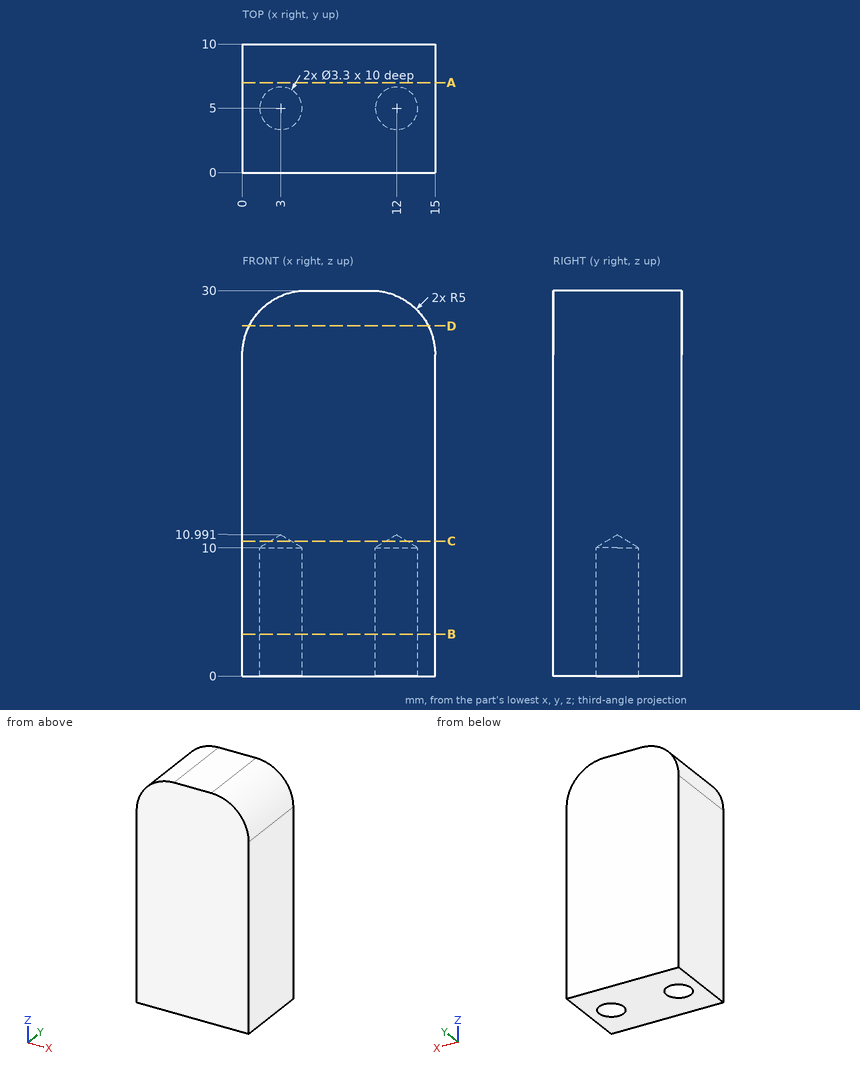
Source: three-view drawing plus pictorial views. Frame: mm from the lowest corner of the part. Coordinates: 2 decimals unless noted, no trailing zeros. Order: outer loops, then holes, each group sorted by start corner. A loop starts at its lowest first (then second) coordinate and runs counter-clockwise, first axis right, second up. Notation, with made-up numbers: (46.25, -27.75) -> (75.25, -27.75) arc R15 ccw to (75.25, -22.75) -> close; hole circle Ø11 at (0.5, 28.5). An arc over 180 degrees is marked (long way). Write item = value, one per line.
(1) Cut plane D-D on z = 27.25. Return loops of the section in (x, y) (1 decimal), plus the area to 3 significant figures.
Solved:
outline = (0.5, 0) -> (14.5, 0) -> (14.5, 10) -> (0.5, 10) -> close
area = 139 mm²
(2) Pin query (flat end, axial travel): pin 1 Ø3 at (x, y) = (3, 8) entering from +Z (1 decimal). Return the tip coordinate at first contact, or that it passes through.
Solved:
pin_1 = 30
(3) Cut plane A-A on y = 7. Return loops of the section in (x, z), plus the area to 3 significant figures.
Solved:
outline = (0, 0) -> (15, 0) -> (15, 25) arc R5 ccw to (10, 30) -> (5, 30) arc R5 ccw to (0, 25) -> close
area = 439 mm²
(4) Cut plane C-C on z = 10.5. Return loops of the section in (x, y) (1 decimal), plus the area to 3 significant figures.
Solved:
outline = (0, 0) -> (15, 0) -> (15, 10) -> (0, 10) -> close; hole circle Ø1.6 at (3, 5); hole circle Ø1.6 at (12, 5)
area = 146 mm²
(5) Cut plane B-B on z = 3.25. Return loops of the section in (x, y), plus the area to 3 significant figures.
Solved:
outline = (0, 0) -> (15, 0) -> (15, 10) -> (0, 10) -> close; hole circle Ø3.3 at (3, 5); hole circle Ø3.3 at (12, 5)
area = 133 mm²
(6) Line query: line 1 (X direction, y = 5, z = 3.75); line 2 (Y direction, x = 12, z = 7.25); line 3 (X direction, y = 4, z = 9.75). Output: solid intervals per line, ascending.
Solved:
line_1 = 0 to 1.35, 4.65 to 10.35, 13.65 to 15
line_2 = 0 to 3.35, 6.65 to 10
line_3 = 0 to 1.69, 4.31 to 10.69, 13.31 to 15
